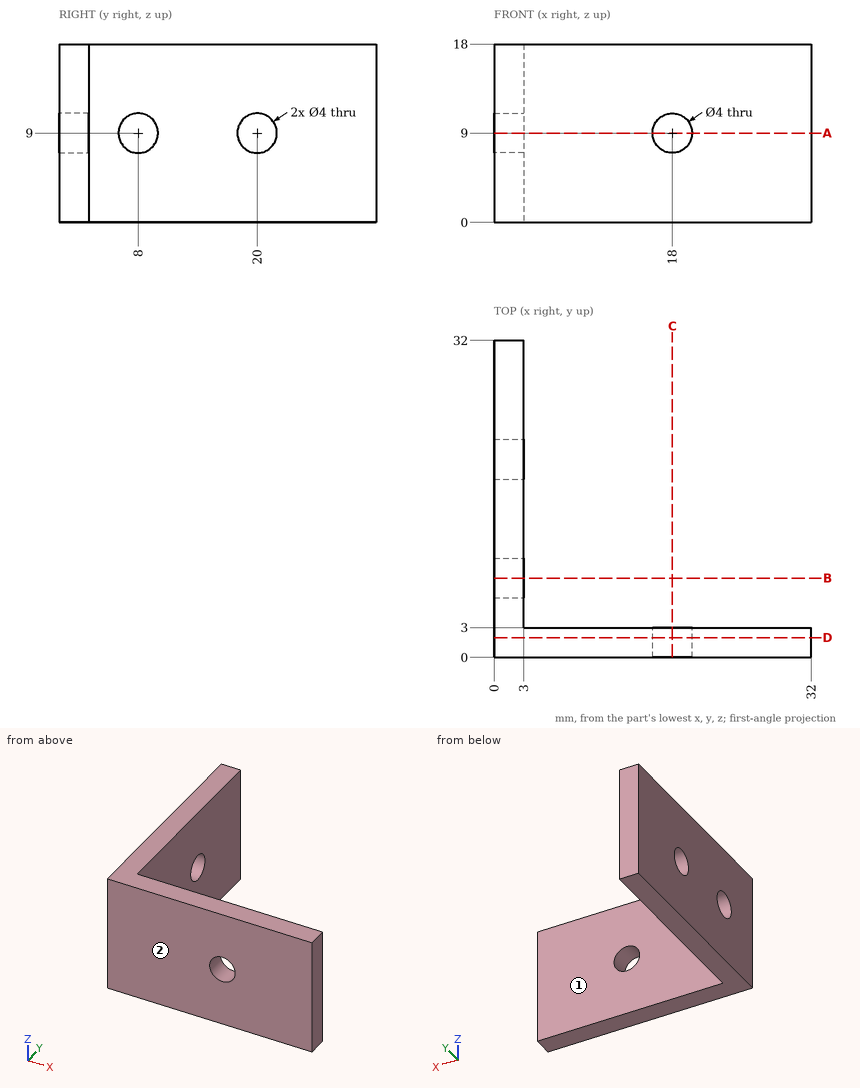
Study the drawing (mm; zero at the part's minimum x, y, z) and answer. A direction names the side the tool comes from. Round coordinates to 2 decimals unless told otherwise and drop trailing zeros. Write each loop counter-clockwise with the first axis right and the second up, starting at its lowest first coordinate (ties: lowest second). Pieces come first, ordered by that corner, then holes.
1) A cutting plane is placed at A-A on z = 9. Determine the outline of the cut face in (x, y), and give its area (3 significant figures).
2) Flat-ended cylindrical pins translate along their axes: P1, Ø4, axis at y = 24.5, z = 2, coming from the +X side; P2, Ø2, axis at x = 10.5, z = 14, coming from the +Y side; P3, Ø2.5, axis at x = 18, z = 9, coming from the -Y side. Find the tip coordinate at first contact, or state that the pin passes through.
3) A cutting plane is placed at D-D on y = 2. Determine the outline of the cut face in (x, z), and give its area (3 significant figures).
4) Consider probe 1 along Y at (x, z) = (1.9, 9); probe 2 along X at (y, z) = (1.25, 9); probe 3 along X at (y, z) = (28, 17). Determine where each line is inside the solid, lowest interval first.
5) A cutting plane is placed at B-B on y = 8. Determine the outline of the cut face in (x, z).
6) Which of the six approach directions +Z, -Z, +X, -X, +Y, -Y give full straight-line access (tool end or side, diameter ignored) to the marked faces 1 and 2?
Entries:
1. outline: (0, 0) - (16, 0) - (16, 3) - (3, 3) - (3, 6) - (0, 6) - close; (0, 10) - (3, 10) - (3, 18) - (0, 18) - close; (0, 22) - (3, 22) - (3, 32) - (0, 32) - close; (20, 0) - (32, 0) - (32, 3) - (20, 3) - close
1. area: 147 mm2
2. P1: stops at x = 3
2. P2: stops at y = 3
2. P3: passes through
3. outline: (0, 0) - (32, 0) - (32, 18) - (0, 18) - close; hole circle Ø4 at (18, 9)
3. area: 563 mm2
4. probe 1: y = 0 to 6, 10 to 18, 22 to 32
4. probe 2: x = 0 to 16, 20 to 32
4. probe 3: x = 0 to 3
5. outline: (0, 0) - (3, 0) - (3, 7) - (0, 7) - close; (0, 11) - (3, 11) - (3, 18) - (0, 18) - close
6. face 1: +Z, -Z, +X, +Y
6. face 2: +Z, -Z, +X, -X, -Y
